Read the model definition and answer for the solid it produces. Units are mm, in the model's axes. A direction names the side the tool comes from. Give positions to 0.01 mm unless a question says otherwise; leave off trailing zeros. Loops run counter-clockwise (first coordinate to the right, second up) from the corner with the lowest first, then second, coordinate; pieces in that order, holes last. Notation, with made-up numbers: (-21, 80.25) - (35, 80.25) arc R27 ccw to (35, 102.25) - close; hole circle Ø7 at (-27.5, 89). An arc over 180 degrees is marked (long way). Put each result on its own line as item: value. Start each with the question number.
1. A cutting plane is placed at C-C, the plane x = 5. Determine the outline of the cut face in (y, z), plus the area to 3 significant figures.
2. Given pin 1 Ø3 at (x, z) = (5.5, -5.5) entering from -Y; pin 2 Ø4 at (x, z) = (9, -8.5) entering from +Y; pin 3 Ø1.5 at (x, z) = (2.5, -3) entering from +Y, each flat-ended and moving along its own axis, determine where each tip first touches the part or whether it passes through.
3. A cutting plane is placed at D-D, the plane y = 10.75. Determine the outline of the cut face in (x, z).
4. Consider L1, parallel to X at y = 6.5, z = -4.5; L2, parallel to Z at x = 4.25, y = 4.75; L3, parallel to Y at x = 13.75, z = -7. Determine where each line is inside the solid, lowest interval first. Write a range as from..to.
5. For a pull along Z with two mould halves and no side action, classify faces 3 (the flat face through (8, 12, -2)), 4 (the flat face through (13, 5, -5)), 5 (the flat face through (8, 13, -7)) as released by +Z, released by -Z, zero draft, split by the parting line, or undercut.
6. A cutting plane is placed at A-A, the plane y = 9. Determine the outline of the cut face in (x, z).
7. A cutting plane is placed at B-B, the plane z = -7. Determine the outline of the cut face in (x, y).
8. For faces 1 (the flat face through (7, 5, -10)), 2 (the flat face through (7, 5, -2)), determine the directions among +Z, -Z, +X, -X, +Y, -Y from which every point of the face is accessible in a straight line to the end or side of a thin tool.
```python
from build123d import *

# Parameters (mm, degrees)
SKETCH1_W           = 15
SKETCH1_H           = 10
SKETCH1_W_2         = 11
SKETCH1_H_2         = 6
BOSS_EXTRUDE1_DEPTH = 10
BOSS_EXTRUDE2_DEPTH = 15


with BuildPart() as part:
    # Sketch1 → Boss-Extrude1 (new body)
    with BuildSketch(Plane(origin=(0, 0, 0), x_dir=(1, 0, 0), z_dir=(0, 1, 0))):
        with Locations((7.5, 5)):
            Rectangle(SKETCH1_W, SKETCH1_H)
        with Locations((7.5, 5)):
            Rectangle(SKETCH1_W_2, SKETCH1_H_2, mode=Mode.SUBTRACT)
    extrude(amount=BOSS_EXTRUDE1_DEPTH)

    # Sketch2 → Boss-Extrude2 (add)
    with BuildSketch(Plane(origin=(15, 0, 0), x_dir=(0, 0, -1), z_dir=(1, 0, 0))):
        Polygon((0, 10), (5, 15), (10, 10), align=None)
    extrude(amount=-BOSS_EXTRUDE2_DEPTH)


solid = part.part
```
Return value:
1. outline: (0, -10) - (10, -10) - (15, -5) - (10, 0) - (0, 0) - (0, -2) - (10, -2) - (10, -8) - (0, -8) - close
1. area: 65.0 mm2
2. pin 1: stops at y = 10
2. pin 2: stops at y = 13.5
2. pin 3: stops at y = 13.75
3. outline: (0, -9.25) - (15, -9.25) - (15, -0.75) - (0, -0.75) - close
4. L1: x = 0..2, 13..15
4. L2: z = -10..-8, -2..0
4. L3: y = 0..13
5. face 3: released by +Z
5. face 4: undercut
5. face 5: released by -Z
6. outline: (0, -10) - (15, -10) - (15, 0) - (0, 0) - close; hole (2, -8) - (13, -8) - (13, -2) - (2, -2) - close
7. outline: (0, 0) - (2, 0) - (2, 10) - (13, 10) - (13, 0) - (15, 0) - (15, 13) - (0, 13) - close
8. face 1: -Z, +X, -X, +Y, -Y
8. face 2: -Y
